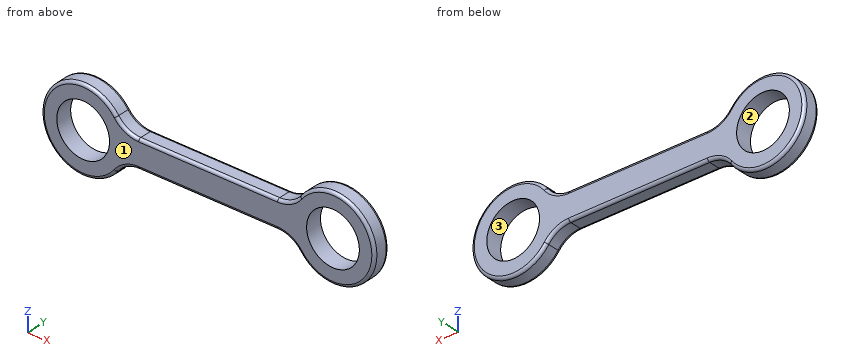
```python
from build123d import *

# Parameters (mm, degrees)
SKETCH1_R           = 9.5
BOSS_EXTRUDE1_DEPTH = 6
FILLET1_R           = 1


with BuildPart() as part:
    # Sketch1 → Boss-Extrude1 (new body)
    with BuildSketch(Plane(origin=(0, 0, 0), x_dir=(1, 0, 0), z_dir=(0, 1, 0))):
        with BuildLine():
            Line((-28.045977011, 5), (21.954022989, 5))
            ThreePointArc((21.954022989, 5), (26.426158944, 6.05572809), (29.954022989, 9))
            ThreePointArc((29.954022989, 9), (56.954022989, 0), (29.954022989, -9))
            ThreePointArc((29.954022989, -9), (26.426158944, -6.05572809), (21.954022989, -5))
            Line((21.954022989, -5), (-28.045977011, -5))
            ThreePointArc((-28.045977011, -5), (-32.518112966, -6.05572809), (-36.045977011, -9))
            ThreePointArc((-36.045977011, -9), (-63.045977011, 0), (-36.045977011, 9))
            ThreePointArc((-36.045977011, 9), (-32.518112966, 6.05572809), (-28.045977011, 5))
        make_face()
        with Locations(Location((-48.045977011, 0, 0), (0, 0, 270))):
            Circle(SKETCH1_R, mode=Mode.SUBTRACT)
        with Locations(Location((41.954022989, 0, 0), (0, 0, 270))):
            Circle(SKETCH1_R, mode=Mode.SUBTRACT)
    extrude(amount=BOSS_EXTRUDE1_DEPTH)

    # Fillet1
    fillet1_edges = [part.edges().sort_by_distance(p)[0] for p in [
        (-63.045977011, 0, 0),
        (-32.518112966, 0, -6.05572809),
        (-3.045977011, 0, -5),
        (26.426158944, 0, -6.05572809),
        (-32.518112966, 6, -6.05572809),
        (-63.045977011, 6, 0),
        (-32.518112966, 6, 6.05572809),
        (-3.045977011, 6, 5),
        (26.426158944, 6, 6.05572809),
        (56.954022989, 6, 0),
        (26.426158944, 6, -6.05572809),
        (56.954022989, 0, 0),
        (-3.045977011, 6, -5),
        (26.426158944, 0, 6.05572809),
        (-3.045977011, 0, 5),
        (-32.518112966, 0, 6.05572809),
    ]]
    fillet(fillet1_edges, radius=FILLET1_R)


solid = part.part
```
Check sheet for the modelled part. Datum: model origin and axes. Units: mm. Face numbers are marked on the shaded views. Give positions to 0.01 mm unless a question says otherwise; leave off trailing zeros. Order: outer loops, then holes, each group sorted by start corner. A loop starts at its lowest first (then second) coordinate and runs counter-clockwise, first axis right, second up. Notation, with made-up numbers: (-18.5, -5.75) -> (14.5, -5.75) arc R21 ccw to (14.5, 2.25) -> close; hole circle Ø5 at (-10, -34.75). An arc over 180 degrees is marked (long way). Return JSON: item names as keys, results as strings.
1. Material ranges on probe 1 along X at (y, z) = (3.4, 0); probe 2 along X at (y, z) = (5, 6); probe 3 along X at (y, z) = (2.6, -4), recorded low to high. Write a range as [from, to].
From the geometry:
{"probe 1": "[-63.05, -57.55], [-38.55, 32.45], [51.45, 56.95]", "probe 2": "[-61.79, -55.41], [-40.68, -32.4], [26.31, 34.59], [49.32, 55.7]", "probe 3": "[-62.5, -56.66], [-39.43, 33.34], [50.57, 56.41]"}
2. Cross-section at C-C, the plane x = -7.5. Record the cut outline in (y, z).
From the geometry:
{"outline": "(0, -4) arc R1 ccw to (1, -5) -> (5, -5) arc R1 ccw to (6, -4) -> (6, 4) arc R1 ccw to (5, 5) -> (1, 5) arc R1 ccw to (0, 4) -> close"}
3. Go/stop test with flat-tipped pins: P1, Ø1, axis at x = -48, z = 7, coming from the +Y side; P2, Ø2, axis at x = -26, y = 4.5, coming from the +Z side; P3, Ø6, axis at x = 39.5, z = 8.5, coming from the +Y side. Record where each tip stops, or that it passes through.
From the geometry:
{"P1": "through", "P2": "z = 5", "P3": "y = 6"}
4. Mould release check, pull along Z, two halves, no side actions. Record for the marked faces 1, 2 and 3: +Z half, -Z half, draft (parallel to the pull), parting line (faces both ways), or undercut.
From the geometry:
{"face 1": "draft", "face 2": "undercut", "face 3": "undercut"}
5. Cross-section at A-A, the plane z = 0. Record the cut outline in (x, y).
From the geometry:
{"outline": "(-63.05, 1) arc R1 ccw to (-62.05, 0) -> (-57.55, 0) -> (-57.55, 6) -> (-62.05, 6) arc R1 ccw to (-63.05, 5) -> close; (-38.55, 0) -> (32.45, 0) -> (32.45, 6) -> (-38.55, 6) -> close; (51.45, 0) -> (55.95, 0) arc R1 ccw to (56.95, 1) -> (56.95, 5) arc R1 ccw to (55.95, 6) -> (51.45, 6) -> close"}
6. Cross-section at B-B, the plane y = 2.1. Record the cut outline in (x, z), plus the area to 3 significant figures.
From the geometry:
{"outline": "(-36.05, -9) arc R10 cw to (-28.05, -5) -> (21.95, -5) arc R10 cw to (29.95, -9) arc R15 ccw (long way) to (29.95, 9) arc R10 cw to (21.95, 5) -> (-28.05, 5) arc R10 cw to (-36.05, 9) arc R15 ccw (long way) to start; hole circle Ø19 at (-48.05, 0); hole circle Ø19 at (41.95, 0)", "area": "1,470 mm^2"}
